from build123d import *

# Parameters (mm, degrees)
BSSXTRD_CLIPTOPFACE_OUTLINE_R   = 1.6764
BSSXTRD_CLIPTOPFACE_OUTLINE_R_2 = 2.159
BSSXTRD_CLIPTOPFACE_DEPTH       = 1.27
SKTCH_CLIPSTANDOFFCROSSSEC_W    = 15.24
SKTCH_CLIPSTANDOFFCROSSSEC_H    = 1.27
BSSXTRD_CLIPLEG_DEPTH           = 11.43
SKTCH_CLIPFOOTCROSSSEC_W        = 15.24
SKTCH_CLIPFOOTCROSSSEC_H        = 1.27
BSSXTRD_CLIPFOOT_DEPTH          = 29.21
CTXTRD_CLIPFOOTHOLES_REACH      = 85.311
SKTCH_CLIPFOOTHOLES_R           = 2.159
SKTCH_CLIPSTANDOFFCROSSSEC_3_W  = 1.27
SKTCH_CLIPSTANDOFFCROSSSEC_3_H  = 25.4
BSSXTRD_CLIPTABS_DEPTH          = 31.75


# Read off the part's stored shape, not the designer's step: BssXtrd_ClipTopFace
with BuildPart() as part:
    # BssXtrd_ClipTopFace outline → BssXtrd_ClipTopFace (new body)
    with BuildSketch(Plane(origin=(0, 0, 0), x_dir=(1, 0, 0), z_dir=(0, 1, 0))):
        Polygon((-7.62, -34.29), (7.62, -34.29), (7.62, 8.89), (52.705, 8.89), (52.705, 34.29), (-52.705, 34.29), (-52.705, 8.89), (-7.62, 8.89), align=None)
        with Locations((0, -26.67)):
            Circle(BSSXTRD_CLIPTOPFACE_OUTLINE_R, mode=Mode.SUBTRACT)
        with Locations((-42.7482, 21.59)):
            Circle(BSSXTRD_CLIPTOPFACE_OUTLINE_R_2, mode=Mode.SUBTRACT)
        with Locations((0, 8.89)):
            Circle(BSSXTRD_CLIPTOPFACE_OUTLINE_R, mode=Mode.SUBTRACT)
        with Locations((42.7482, 21.59)):
            Circle(BSSXTRD_CLIPTOPFACE_OUTLINE_R_2, mode=Mode.SUBTRACT)
    extrude(amount=BSSXTRD_CLIPTOPFACE_DEPTH)

    # Sktch_ClipStandoffCrossSec → BssXtrd_ClipLeg (add)
    with BuildSketch(Plane.XZ):
        with Locations((0, 33.655)):
            Rectangle(SKTCH_CLIPSTANDOFFCROSSSEC_W, SKTCH_CLIPSTANDOFFCROSSSEC_H)
    extrude(amount=BSSXTRD_CLIPLEG_DEPTH)

    # Sktch_ClipFootCrossSec → BssXtrd_ClipFoot (add)
    with BuildSketch(Plane.XY.offset(34.29)):
        with Locations((0, -10.795)):
            Rectangle(SKTCH_CLIPFOOTCROSSSEC_W, SKTCH_CLIPFOOTCROSSSEC_H)
    extrude(amount=BSSXTRD_CLIPFOOT_DEPTH)

    # Sktch_ClipFootHoles → CtXtrd_ClipFootHoles (cut, up to next)
    with BuildSketch(Plane(origin=(0, -10.16, 0), x_dir=(1, 0, 0), z_dir=(0, 1, 0)), mode=Mode.PRIVATE) as ctxtrd_clipfootholes_sk1:
        with Locations(Location((0, -42.418, 0), (0, 0, 180))):
            Circle(SKTCH_CLIPFOOTHOLES_R)
    ctxtrd_clipfootholes_tool1 = extrude(ctxtrd_clipfootholes_sk1.sketch, amount=-CTXTRD_CLIPFOOTHOLES_REACH, mode=Mode.PRIVATE) & part.part
    # Sktch_ClipFootHoles → CtXtrd_ClipFootHoles (cut, up to next)
    with BuildSketch(Plane(origin=(0, -10.16, 0), x_dir=(1, 0, 0), z_dir=(0, 1, 0)), mode=Mode.PRIVATE) as ctxtrd_clipfootholes_sk2:
        with Locations(Location((0, -57.4802, 0), (0, 0, 180))):
            Circle(SKTCH_CLIPFOOTHOLES_R)
    ctxtrd_clipfootholes_tool2 = extrude(ctxtrd_clipfootholes_sk2.sketch, amount=-CTXTRD_CLIPFOOTHOLES_REACH, mode=Mode.PRIVATE) & part.part
    add(ctxtrd_clipfootholes_tool1.solids().sort_by_distance((0, -10.16, 42.418))[0], mode=Mode.SUBTRACT)
    add(ctxtrd_clipfootholes_tool2.solids().sort_by_distance((0, -10.16, 57.4802))[0], mode=Mode.SUBTRACT)

    # Sktch_ClipStandoffCrossSec<3> → BssXtrd_ClipTabs (add)
    with BuildSketch(Plane.XZ):
        with Locations((52.07, -21.59)):
            Rectangle(SKTCH_CLIPSTANDOFFCROSSSEC_3_W, SKTCH_CLIPSTANDOFFCROSSSEC_3_H)
        with Locations((-52.07, -21.59)):
            Rectangle(SKTCH_CLIPSTANDOFFCROSSSEC_3_W, SKTCH_CLIPSTANDOFFCROSSSEC_3_H)
    extrude(amount=BSSXTRD_CLIPTABS_DEPTH)


solid = part.part
Design review of the part built by this model. Coordinates are the model's own, in mm. A direction names the side the tool comes from. Round coordinates to 2 decimals unless told otherwise and drop trailing zeros. Loops run counter-clockwise (first coordinate to the right, second up) from the corner with the lowest first, then second, coordinate; pieces in that order, holes last. Notation, with made-up numbers: M 32.25,-14 L 81.25,-14 A31 ccw 81.25,21 Z; hole C 87,-27 d6. An arc over 180 degrees is marked long. Answer as a JSON object with one key per item and string values.
Item 1: We need section A-A on x = 0. Give the boundary of the cut face in (y, z), and give its area (3 significant figures).
Answer sheet:
{"outline": "M -11.43,33.02 L 0,33.02 L 0,28.35 L 1.27,28.35 L 1.27,34.29 L -10.16,34.29 L -10.16,40.26 L -11.43,40.26 Z; M -11.43,44.58 L -10.16,44.58 L -10.16,55.32 L -11.43,55.32 Z; M -11.43,59.64 L -10.16,59.64 L -10.16,63.5 L -11.43,63.5 Z; M 0,-34.29 L 1.27,-34.29 L 1.27,-10.57 L 0,-10.57 Z; M 0,-7.21 L 1.27,-7.21 L 1.27,24.99 L 0,24.99 Z", "area": "119 mm^2"}
Item 2: The part is to be moulded in two halves that separate along Y. For faces 1 (the flat face through (-1, 1.27, -16)), 2 (the flat face through (-1, 0, -16)), 3 (the cylindrical face through (42.47, 0.63, -23.73)), say which applies: pulls with the +Y half, pulls with the -Y half, needs draft (parallel to the pull), parting line crosses it, or undercut.
Answer sheet:
{"face 1": "pulls with the +Y half", "face 2": "pulls with the -Y half", "face 3": "needs draft"}
Item 3: Wall thickness on L1, parallel to Z at x = 0, y = 0.7; L2, parallel to X at y = -21.5, z = -11 (3 decimals); L3, parallel to X at y = -10.5, z = 54: over which ranges is each line inside the solid? List them lowest first. Write a range as from..to.
Answer sheet:
{"L1": "z = -34.29..-10.57, -7.21..24.99, 28.35..34.29", "L2": "x = -52.705..-51.435, 51.435..52.705", "L3": "x = -7.62..7.62"}
Item 4: We need section B-B on y = -27.5. Give the boundary of the cut face in (x, z) (3 decimals), and give its area (3 significant figures).
Answer sheet:
{"outline": "M -52.705,-34.29 L -51.435,-34.29 L -51.435,-8.89 L -52.705,-8.89 Z; M 51.435,-34.29 L 52.705,-34.29 L 52.705,-8.89 L 51.435,-8.89 Z", "area": "64.5 mm^2"}
Item 5: Machinability: for faces 4 (the flat face through (-40, 1, -8.89)), 5 (the flat face through (51.435, -16, -22)), 6 (the flat face through (0, -6, 33.02)), 7 (the flat face through (40, 1, -8.89)), 8 (the flat face through (0, -4, 34.29)), which of the approach directions +Z, -Z, +X, -X, +Y, -Y give a long, thin tool a straight path to every point of the face, cutting with its end or side? Answer none if there is none.
Answer sheet:
{"face 4": "+Z, -X, +Y, -Y", "face 5": "+Z, -Z, -Y", "face 6": "-Z, +X, -X, -Y", "face 7": "+Z, +X, +Y, -Y", "face 8": "+Z, +X, -X, +Y"}
Item 6: We need section C-C on y = -6. Give the boundary of the cut face in (x, z) (3 decimals).
Answer sheet:
{"outline": "M -52.705,-34.29 L -51.435,-34.29 L -51.435,-8.89 L -52.705,-8.89 Z; M -7.62,33.02 L 7.62,33.02 L 7.62,34.29 L -7.62,34.29 Z; M 51.435,-34.29 L 52.705,-34.29 L 52.705,-8.89 L 51.435,-8.89 Z"}
Item 7: Clearance check with flat-ended pins moving along their axes: P1, Ø7.5, axis at x = -2.5, z = 55.5, coming from the -Y side; P2, Ø7, axis at x = -42.75, z = -21.59, coming from the -Y side; P3, Ø5, axis at y = -9, z = 29, coming from the -X side; P4, Ø5.5, axis at x = 1.5, y = -3.5, coming from the -Z side. State where each tip first meets the part, or that it passes through.
Answer sheet:
{"P1": "stops at y = -11.43", "P2": "stops at y = 0", "P3": "passes through", "P4": "stops at z = 33.02"}
Item 8: We need section D-D on z = -21.59. Give the boundary of the cut face in (x, y) (3 decimals), and give its area (3 significant figures).
Answer sheet:
{"outline": "M -52.705,-31.75 L -51.435,-31.75 L -51.435,0 L -44.907,0 L -44.907,1.27 L -52.705,1.27 Z; M -40.589,0 L 40.589,0 L 40.589,1.27 L -40.589,1.27 Z; M 44.907,0 L 51.435,0 L 51.435,-31.75 L 52.705,-31.75 L 52.705,1.27 L 44.907,1.27 Z", "area": "204 mm^2"}
